Read the model definition and answer for the solid it produces. Units are mm, in the model's axes. Face numbers are marked on the shaded views. A direction names the side the tool comes from. Give positions to 0.01 mm unless a question says otherwise; leave off trailing zeros. Write each loop counter-clockwise with the first axis right and the second up, starting at its lowest first coordinate (ties: lowest second). Pieces come first, ordered by that corner, then holes. Notation, with made-up numbers: (-39.5, -31) - (16.5, -31) arc R31 cw to (16.5, 0) - close; hole circle Ø8 at (53, -12.75). An arc over 180 degrees is marked (long way). Answer as CSV lines item,"result".
```python
from build123d import *

# Parameters (mm, degrees)
SKETCH1_R               = 50
SKETCH1_R_2             = 40
BOSS_EXTRUDE1_DEPTH     = 12
SKETCH1_4_R             = 7.5
SKETCH1_4_R_2           = 4
BOSS_EXTRUDE2_DEPTH     = 16.5
BOSS_EXTRUDE3_START     = 3.5
SKETCH1_5_R             = 40
SKETCH1_5_R_2           = 7.5
BOSS_EXTRUDE3_DEPTH     = 4
SKETCH2_R               = 15
SKETCH2_R_2             = 6
CUT_EXTRUDE3_DEPTH      = 17.5
CUT_EXTRUDE3_DEPTH_BACK = 1
SKETCH3_R               = 1.5
CUT_EXTRUDE4_DEPTH      = 10
CUT_EXTRUDE4_DEPTH_BACK = 10


with BuildPart() as part:
    # Sketch1 → Boss-Extrude1 (new body)
    with BuildSketch(Plane(origin=(0, 0, 0), x_dir=(1, 0, 0), z_dir=(0, 1, 0))):
        Circle(SKETCH1_R)
        Circle(SKETCH1_R_2, mode=Mode.SUBTRACT)
    extrude(amount=BOSS_EXTRUDE1_DEPTH)



with BuildPart() as body_2:
    # Sketch1<4> → Boss-Extrude2 (new body)
    with BuildSketch(Plane(origin=(0, 0, 0), x_dir=(1, 0, 0), z_dir=(0, 1, 0))):
        Circle(SKETCH1_4_R)
        Circle(SKETCH1_4_R_2, mode=Mode.SUBTRACT)
    extrude(amount=BOSS_EXTRUDE2_DEPTH)


with BuildPart() as part_1:
    add(part.part)

    add(body_2.part)  # Boss-Extrude3 merges body 2
    # Sketch1<5> → Boss-Extrude3 (add)
    with BuildSketch(Plane(origin=(0, 0, 0), x_dir=(1, 0, 0), z_dir=(0, 1, 0)).offset(BOSS_EXTRUDE3_START)):
        Circle(SKETCH1_5_R)
        Circle(SKETCH1_5_R_2, mode=Mode.SUBTRACT)
    extrude(amount=BOSS_EXTRUDE3_DEPTH)

    # Sketch2 → Cut-Extrude3 (cut, two sides)
    with BuildSketch(Plane(origin=(0, 0, 0), x_dir=(1, 0, 0), z_dir=(0, 1, 0))) as cut_extrude3_sk:
        with Locations((-23.75, 0)):
            Circle(SKETCH2_R)
        with Locations((0, -23.75)):
            Circle(SKETCH2_R)
        with Locations((-22.627416998, -22.627416998)):
            Circle(SKETCH2_R_2)
        with Locations((-22.627416998, 22.627416998)):
            Circle(SKETCH2_R_2)
        with Locations((0, 23.75)):
            Circle(SKETCH2_R)
        with Locations((23.75, 0)):
            Circle(SKETCH2_R)
        with Locations((22.627416998, -22.627416998)):
            Circle(SKETCH2_R_2)
        with Locations((22.627416998, 22.627416998)):
            Circle(SKETCH2_R_2)
    extrude(amount=CUT_EXTRUDE3_DEPTH, mode=Mode.SUBTRACT)
    extrude(cut_extrude3_sk.sketch, amount=-CUT_EXTRUDE3_DEPTH_BACK, mode=Mode.SUBTRACT)

    # Sketch3 → Cut-Extrude4 (cut, two sides)
    with BuildSketch(Plane.XY) as cut_extrude4_sk:
        with Locations((0, 13)):
            Circle(SKETCH3_R)
    extrude(amount=CUT_EXTRUDE4_DEPTH, mode=Mode.SUBTRACT)
    extrude(cut_extrude4_sk.sketch, amount=-CUT_EXTRUDE4_DEPTH_BACK, mode=Mode.SUBTRACT)


solid = part_1.part
```
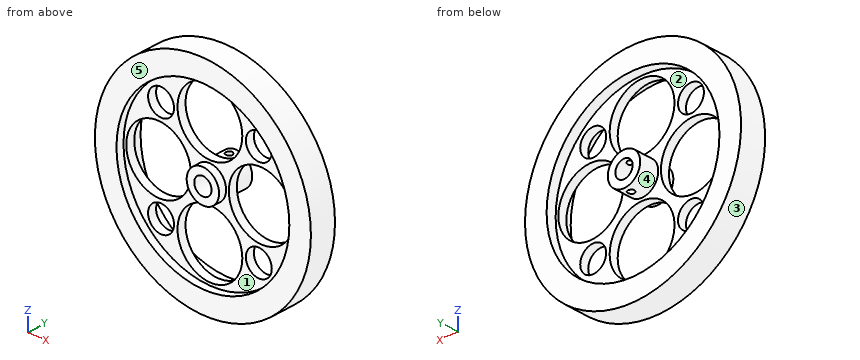
(1) A cutting plane is placed at B-B (x = 31). Write down the section's boundary in (y, z).
Worked out:
outline,"(0, -39.23) - (12, -39.23) - (12, -25.28) - (7.5, -25.28) - (7.5, -13.13) - (3.5, -13.13) - (3.5, -25.28) - (0, -25.28) - close; (0, 25.28) - (3.5, 25.28) - (3.5, 13.13) - (7.5, 13.13) - (7.5, 25.28) - (12, 25.28) - (12, 39.23) - (0, 39.23) - close"
(2) A cutting plane is placed at A-A (z = 0). Count the separate pieces of the cut face and the enclosed holes in it, and give its area (4 significant figures).
Worked out:
separate pieces,"4"
enclosed holes,"0"
area,"375.5 mm^2"
(3) The mould has two halves that part along Z. Classify the marked faces 3, 4 and 5: +Z half, -Z half, draft (parallel to the pull), parting line (faces both ways), or undercut.
Worked out:
face 3,"parting line"
face 4,"undercut"
face 5,"draft"
(4) Find the intervals of material crossed by L1, parallel to X at y = 0.9, z = 0; L2, parallel to Z at x = -23.75, y = 5.4; L3, parallel to Z at x = 0, y = 6, in increasing order.
Worked out:
L1,"x = -50 to -40, -7.5 to -4, 4 to 7.5, 40 to 50"
L2,"z = -44 to -28.52, -16.73 to -15, 15 to 16.73, 28.52 to 44"
L3,"z = -50 to -38.75, -8.75 to -4, 4 to 8.75, 38.75 to 50"
(5) For the marked faces 1 and 2, determine the directions among +Z, -Z, +X, -X, +Y, -Y from which every point of the face is accessible in a straight line to the end or side of a thin tool.
Worked out:
face 1,"-Y"
face 2,"+Y"
(6) A cutting plane is placed at C-C (x = -12). Write down the section's boundary in (y, z).
Worked out:
outline,"(0, -48.54) - (12, -48.54) - (12, -38.16) - (7.5, -38.16) - (7.5, -32.75) - (3.5, -32.75) - (3.5, -38.16) - (0, -38.16) - close; (0, 38.16) - (3.5, 38.16) - (3.5, 32.75) - (7.5, 32.75) - (7.5, 38.16) - (12, 38.16) - (12, 48.54) - (0, 48.54) - close; (3.5, -14.75) - (7.5, -14.75) - (7.5, -9.32) - (3.5, -9.32) - close; (3.5, 9.32) - (7.5, 9.32) - (7.5, 14.75) - (3.5, 14.75) - close"
(7) Each of these flat-tipped pins is pushed along its axis until it touches: P1, Ø1.5, axis at x = -31, z = -24, coming from the +Y side; P2, Ø6, axis at y = 13.5, z = 39, coming from the -X side; P3, Ø9.5, axis at x = -22.63, z = 22.63, coming from the +Y side; P4, Ø5, axis at x = 0, y = 13, coming from the +Z side. Where does it stop, or does it pass through?
Worked out:
P1,"stops at y = 7.5"
P2,"stops at x = -34.28"
P3,"passes through"
P4,"stops at z = 50"
